from build123d import *

# Parameters (mm, degrees)
SKETCH1_R           = 17.5
SKETCH1_R_2         = 12.7
BOSS_EXTRUDE1_DEPTH = 5
SKETCH2_R           = 22.5
SKETCH2_R_2         = 12.7
BOSS_EXTRUDE2_DEPTH = 2
SKETCH3_R           = 1.6
CUT_EXTRUDE1_DEPTH  = 23.5
CUT_EXTRUDE2_DEPTH  = 23.5
SKETCH5_R           = 2.75
CUT_EXTRUDE3_DEPTH  = 8.5


with BuildPart() as part:
    # Sketch1 → Boss-Extrude1 (new body, symmetric)
    with BuildSketch(Plane(origin=(0, 0, 0), x_dir=(1, 0, 0), z_dir=(0, 1, 0))):
        Circle(SKETCH1_R)
        Circle(SKETCH1_R_2, mode=Mode.SUBTRACT)
    extrude(amount=BOSS_EXTRUDE1_DEPTH, both=True)

    # Sketch2 → Boss-Extrude2 (add)
    with BuildSketch(Plane(origin=(0, 5, 0), x_dir=(1, 0, 0), z_dir=(0, 1, 0))):
        Circle(SKETCH2_R)
        Circle(SKETCH2_R_2, mode=Mode.SUBTRACT)
    boss_extrude2 = extrude(amount=BOSS_EXTRUDE2_DEPTH)

    # Mirror1: Boss-Extrude2 across plane
    add(boss_extrude2.mirror(Plane.ZX))

    # Sketch3 → Cut-Extrude1 (cut, through all)
    with BuildSketch(Plane(origin=(0, 0, 0), x_dir=(0, 0, -1), z_dir=(1, 0, 0))):
        Circle(SKETCH3_R)
    extrude(amount=-CUT_EXTRUDE1_DEPTH, mode=Mode.SUBTRACT)

    # Sketch4 → Cut-Extrude2 (cut, through all)
    with BuildSketch(Plane(origin=(0, 0, 0), x_dir=(0, 0, -1), z_dir=(1, 0, 0))):
        Polygon((3.175426481, 0), (1.58771324, 2.75), (-1.58771324, 2.75), (-3.175426481, 0), (-1.58771324, -2.75), (1.58771324, -2.75), align=None)
    extrude(amount=CUT_EXTRUDE2_DEPTH, mode=Mode.SUBTRACT)

    # Sketch5 → Cut-Extrude3 (cut, through all)
    with BuildSketch(Plane(origin=(-15, 0, 0), x_dir=(0, 0, -1), z_dir=(1, 0, 0))):
        Circle(SKETCH5_R)
    extrude(amount=-CUT_EXTRUDE3_DEPTH, mode=Mode.SUBTRACT)


solid = part.part
For this review, take the finished solid that the model builds, in its own axes (mm). A direction names the side the tool comes from. Give positions to 0.01 mm unless a question says otherwise; leave off trailing zeros. Order: outer loops, then holes, each group sorted by start corner. A loop starts at its lowest first (then second) coordinate and runs counter-clockwise, first axis right, second up. Notation, with made-up numbers: (57.25, 56) - (113.25, 56) arc R8 cw to (113.25, 60) - close; hole circle Ø1 at (80, 78.5). An arc over 180 degrees is marked (long way). Answer as a JSON object with one key per item and string values. Group by question number.
Item 1: Machinability: for faces 5 (the cylindrical face through (-13.78, -0.97, 1.27)), 6 (the flat face through (-15, 0, -2)), 7 (the cylindrical face through (16.166, 0.07, 6.703)), 8 (the cylindrical face through (10.382, -5.986, 19.961)), 9 (the flat face through (14.826, 1.394, 2.37)), which of the approach directions +Z, -Z, +X, -X, +Y, -Y give a long, thin tool a straight path to every point of the face, cutting with its end or side? Answer none if there is none.
Item 2: Take a section at B-B on z = 0. Give the boundary of the cut face in (x, y).
Item 3: Take a section at D-D on y = 5.75. Give the boundary of the cut face in (x, z), and give its area (3 significant figures).
Item 4: Draft analysis for pull direction Y (two halves, no side actions). For faces 1 (the flat face through (10, -7, 10)), 2 (the cylindrical face through (10.382, 5.986, 19.961)), 3 (the flat face through (10, 7, 10)), 4 (the cylindrical face through (-16.235, 0.121, 2.747)), state which applies: pulls with the +Y half, pulls with the -Y half, needs draft (parallel to the pull), parting line crosses it, or undercut.
Item 5: Take a section at C-C on z = 9. Give the boundary of the cut face in (x, y), and give its area (3 significant figures).
Item 6: Take a section at A-A on x = 0. Give the boundary of the cut face in (y, z).
Item 7: Wall thickness on line 1 along Y through (x, z) = (-11.5, 19); line 2 along Y through (x, z) = (-16.9, 0); line 3 along Z through (x, y) = (0, 4): over which ranges is each line inside the solid? List them lowest first.
Item 8: Clearance check with flat-ended pins moving along their axes: pin 1 Ø1 at (x, y) = (-5.5, 0) entering from +Z; pin 2 Ø1.5 at (x, y) = (-16, 4.5) entering from -Z; pin 3 Ø3.5 at (y, z) = (0, 0) entering from +X. State where each tip first meets the part, or that it passes through.
Reported:
{
 "1": {"face 5": "+X, -X", "face 6": "-X", "face 7": "none", "face 8": "+Y, -Y", "face 9": "+X"},
 "2": {"outline": "(-22.5, -7) - (-12.7, -7) - (-12.7, -1.6) - (-15, -1.6) - (-15, -2.75) - (-17.5, -2.75) - (-17.5, -5) - (-22.5, -5) - close; (-22.5, 5) - (-17.5, 5) - (-17.5, 2.75) - (-15, 2.75) - (-15, 1.6) - (-12.7, 1.6) - (-12.7, 7) - (-22.5, 7) - close; (12.7, -7) - (22.5, -7) - (22.5, -5) - (17.5, -5) - (17.5, -2.75) - (12.7, -2.75) - close; (12.7, 2.75) - (17.5, 2.75) - (17.5, 5) - (22.5, 5) - (22.5, 7) - (12.7, 7) - close"},
 "3": {"outline": "circle Ø45 at (0, 0); hole circle Ø25.4 at (0, 0)", "area": "1,080 mm^2"},
 "4": {"face 1": "pulls with the -Y half", "face 2": "needs draft", "face 3": "pulls with the +Y half", "face 4": "undercut"},
 "5": {"outline": "(-20.62, -7) - (-8.96, -7) - (-8.96, 7) - (-20.62, 7) - (-20.62, 5) - (-15.01, 5) - (-15.01, -5) - (-20.62, -5) - close; (8.96, -7) - (20.62, -7) - (20.62, -5) - (15.01, -5) - (15.01, 5) - (20.62, 5) - (20.62, 7) - (8.96, 7) - close", "area": "214 mm^2"},
 "6": {"outline": "(-7, -22.5) - (-5, -22.5) - (-5, -17.5) - (5, -17.5) - (5, -22.5) - (7, -22.5) - (7, -12.7) - (-7, -12.7) - close; (-7, 12.7) - (7, 12.7) - (7, 22.5) - (5, 22.5) - (5, 17.5) - (-5, 17.5) - (-5, 22.5) - (-7, 22.5) - close"},
 "7": {"line 1": "-7 to -5, 5 to 7", "line 2": "-7 to -2.75, 2.75 to 7", "line 3": "-17.5 to -12.7, 12.7 to 17.5"},
 "8": {"pin 1": "z = 16.77", "pin 2": "z = -16.37", "pin 3": "x = -12.58"}
}
